Autodesk Inventor part; units mm, degrees
ref_plane "YZ Plane" through (0, 0, 0) normal (1, 0, 0) x (0, 1, 0)
ref_plane "XZ Plane" through (0, 0, 0) normal (0, 1, 0) x (-1, 0, 0)
ref_plane "XY Plane" through (0, 0, 0) normal (0, 0, 1) x (1, 0, 0)
sketch "草图1" plane through (0, 0, 0) normal (1, 0, 0) x (0, 1, 0)
  circle A0 centre (0, 0) radius 5
  dimension "d0" = 10
extrude "拉伸1" add sketch "草图1" along normal blind 15
sketch "草图2" plane through (15, 0, 0) normal (1, 0, 0) x (0, 0, -1)
  line L0 (10, 10) -> (-10, 10)
  line L1 (-10, 10) -> (-10, -10)
  line L2 (-10, -10) -> (10, -10)
  line L3 (10, -10) -> (10, 10)
  point P0 (0, 0)
  dimension "d3" = 20
  dimension "d4" = 20
extrude "拉伸2" add sketch "草图2" along normal blind 2
sketch "草图3" plane through (0, 0, 0) normal (-1, 0, 0) x (0, 0, 1)
  circle A0 centre (0, 0) radius 5
extrude "拉伸3" add sketch "草图3" along normal blind 10
properties part number "激光传感器"
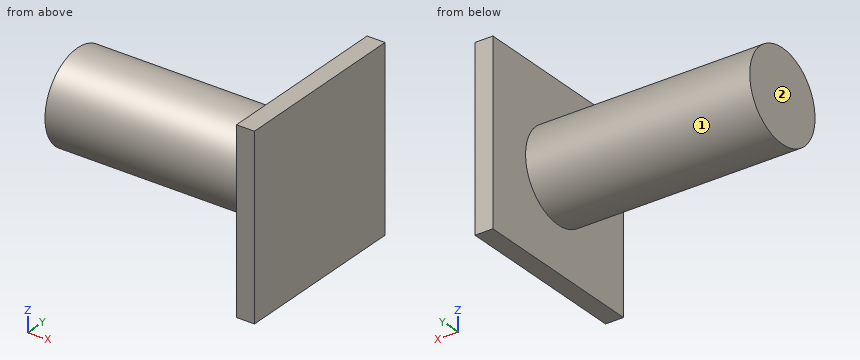
Work out the finished part from the listing and answer in its coordinate system (mm). Face numbers are marked on the shaded views. A direction names the side the tool comes from. Coordinates: 2 decimals unless noted, no trailing zeros. Order: outer loops, then holes, each group sorted by start corner. A loop starts at its lowest first (then second) coordinate and runs counter-clockwise, first axis right, second up. Notation, with made-up numbers: M 25.25,77 L 66.25,77 A14 ccw 66.25,89 Z; hole C -20.5,65 d3. An arc over 180 degrees is marked long. Use CSV: the item, a comma, the result in double quotes.
1) Flat-ended cylindrical pins translate along their axes: pin 1 Ø10 at (x, y) = (5.5, -4) entering from +Z; pin 2 Ø6 at (x, y) = (1.5, -2.5) entering from -Z; pin 3 Ø3 at (x, y) = (12.5, 3.5) entering from -Z. Find the tip coordinate at first contact, or state that the pin passes through.
Worked out:
pin 1,"stops at z = 5"
pin 2,"stops at z = -5"
pin 3,"stops at z = -4.58"
2) Section D-D on y = 8.25 is taken. Write down the section's boundary in (x, z).
Worked out:
outline,"M 15,-10 L 17,-10 L 17,10 L 15,10 Z"
3) Section C-C on z = -2.75 is taken. Write down the section's boundary in (x, y).
Worked out:
outline,"M -10,-4.18 L 15,-4.18 L 15,-10 L 17,-10 L 17,10 L 15,10 L 15,4.18 L -10,4.18 Z"
4) Section B-B on x = -2.5 is taken. Write down the section's boundary in (y, z), plus the area to 3 significant figures.
Worked out:
outline,"C 0,0 d10"
area,"78.5 mm^2"
5) Consider line 1 (X direction, y = 7.5, z = -9); line 2 (Z direction, x = 11, y = -0.25); line 3 (Y direction, x = -6, z = -1.75). Determine where each line is inside the solid, lowest interval first. Write a range as [from, to].
Worked out:
line 1,"x = [15, 17]"
line 2,"z = [-4.99, 4.99]"
line 3,"y = [-4.68, 4.68]"
6) For the marked faces 1 and 2, determine the directions among +Z, -Z, +X, -X, +Y, -Y from which every point of the face is accessible in a straight line to the end or side of a thin tool.
Worked out:
face 1,"-X"
face 2,"+Z, -Z, -X, +Y, -Y"
7) Section A-A on y = -4 is taken. Write down the section's boundary in (x, z).
Worked out:
outline,"M -10,-3 L 15,-3 L 15,-10 L 17,-10 L 17,10 L 15,10 L 15,3 L -10,3 Z"
